Design review of the part built by this model. Coordinates are the model's own, in mm. Give positions to 0.01 mm unless a question says otherwise; leave off trailing zeros. Loops run counter-clockwise (first coordinate to the right, second up) from the corner with the lowest first, then second, coordinate; pieces in that order, holes last. Notation, with made-up numbers: (-18.75, 12) -> (-13.75, 12) arc R13 cw to (-13.75, 36) -> close; hole circle Ø11 at (72, 25). An arc over 180 degrees is marked (long way). Answer as CSV lines item,"result".
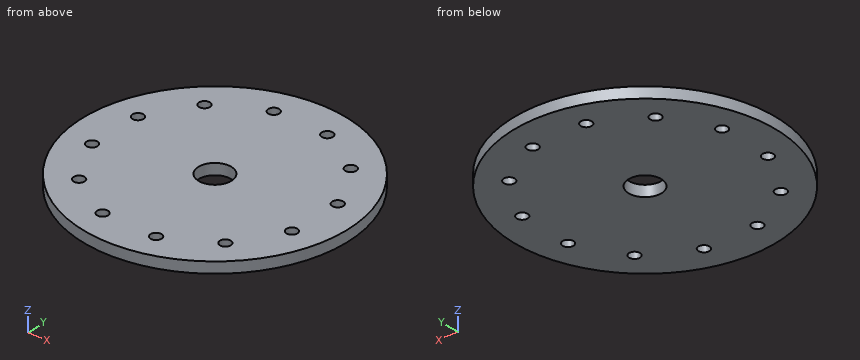
from build123d import *

# Parameters (mm, degrees)
SKETCH1_R           = 152.4
SKETCH1_R_2         = 19.05
BOSS_EXTRUDE1_DEPTH = 12.7
SKETCH2_R           = 6.35
CUT_EXTRUDE2_DEPTH  = 216.9
CRVPATTERN1_COUNT   = 12


with BuildPart() as part:
    # Sketch1 → Boss-Extrude1 (new body)
    with BuildSketch(Plane.XY):
        Circle(SKETCH1_R)
        Circle(SKETCH1_R_2, mode=Mode.SUBTRACT)
    extrude(amount=BOSS_EXTRUDE1_DEPTH)

    # Sketch2 → Cut-Extrude2 (cut, symmetric)
    with BuildSketch(Plane.XY):
        with Locations((85.31243315, 85.31243315)):
            Circle(SKETCH2_R)
    cut_extrude2 = extrude(amount=CUT_EXTRUDE2_DEPTH, both=True, mode=Mode.SUBTRACT)

    # CrvPattern1: Cut-Extrude2 ×12 about axis
    crvpattern1_axis = Axis((0, 0, 0), (0, 0, 1))
    for i in range(1, CRVPATTERN1_COUNT):
        add(cut_extrude2.rotate(crvpattern1_axis, i * 360 / CRVPATTERN1_COUNT), mode=Mode.SUBTRACT)


solid = part.part
Q1. We need section C-C, the plane z = 3.5. State how many separate pieces and enclosed holes the cut face has, and give its area (3 significant figures).
Filled sheet:
separate pieces,"1"
enclosed holes,"13"
area,"70,300 mm^2"
Q2. Clearance check with flat-ended pins moving along their axes: pin 1 Ø2 at (y, z) = (119.5, 9.5) entering from -X; pin 2 Ø11.5 at (x, y) = (31.23, -116.54) entering from +Z; pin 3 Ø1 at (y, z) = (-76, 2.5) entering from -X; pin 4 Ø1.5 at (x, z) = (-109.5, 9.5) entering from +Y. State where each tip first meets the part, or that it passes through.
Filled sheet:
pin 1,"stops at x = -95.83"
pin 2,"passes through"
pin 3,"stops at x = -132.38"
pin 4,"stops at y = 106.77"
Q3. We need section A-A, the plane y = 0. State the section outline as (x, z) points, and give its area (3 significant figures).
Filled sheet:
outline,"(-152.4, 0) -> (-19.05, 0) -> (-19.05, 12.7) -> (-152.4, 12.7) -> close; (19.05, 0) -> (152.4, 0) -> (152.4, 12.7) -> (19.05, 12.7) -> close"
area,"3,390 mm^2"
Q4. We need section D-D, the plane x = 61. State the section outline as (y, z) points, and give its area (3 significant figures).
Filled sheet:
outline,"(-139.66, 0) -> (139.66, 0) -> (139.66, 12.7) -> (-139.66, 12.7) -> close"
area,"3,550 mm^2"
Q5. To check wall thickness, follow probe 1 along X at (y, z) = (-31.5, 6.25); probe 2 along Y at (x, z) = (36.5, 8.5); probe 3 along X at (y, z) = (-85, 4). State the ranges of each line that lie inside material, in increasing order. Write a range as from..to.
Filled sheet:
probe 1,"x = -149.11..-122.88, -110.19..110.19, 122.88..149.11"
probe 2,"y = -147.96..-120.08, -113..113, 120.08..147.96"
probe 3,"x = -126.49..-91.65, -78.97..78.97, 91.65..126.49"
